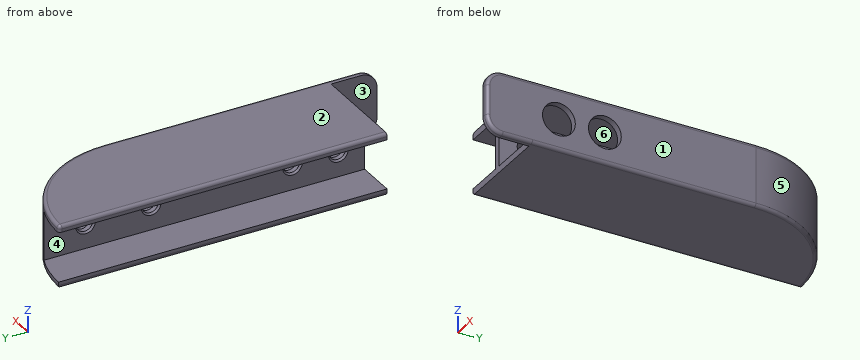
from build123d import *

# Parameters (mm, degrees)
BOSS_EXTRUDE1_DEPTH = 19
SKETCH2_W           = 24
SKETCH2_H           = 15
CUT_EXTRUDE1_DEPTH  = 29
SKETCH2_2_W         = 24
SKETCH2_2_H         = 15
CUT_EXTRUDE2_DEPTH  = 109
SHELL2_START        = 2
SHELL2_DEPTH        = 15
FILLET1_R           = 1
SKETCH8_W           = 2
SKETCH8_H           = 19
BOSS_EXTRUDE2_DEPTH = 14
FILLET3_R           = 5
FILLET4_R           = 1


# Read off the part's stored shape, not the designer's step: Shell2, M6 Tapped Hole1, Ø10.0mm Dowel Hole1
with BuildPart() as part:
    # Sketch1 → Boss-Extrude1 (new body)
    with BuildSketch(Plane.XY):
        with BuildLine():
            Line((32, 0), (32, 68))
            ThreePointArc((32, 68), (22.627416998, 90.627416998), (0, 100))
            Line((0, 100), (0, 0))
            Line((0, 0), (32, 0))
        make_face()
    extrude(amount=BOSS_EXTRUDE1_DEPTH)

    # Sketch2 → Cut-Extrude1 (cut)
    with BuildSketch(Plane(origin=(0, 0, 0), x_dir=(1, 0, 0), z_dir=(0, 1, 0))):
        with Locations((0, -9.5)):
            Rectangle(SKETCH2_W, SKETCH2_H)
    extrude(amount=CUT_EXTRUDE1_DEPTH, mode=Mode.SUBTRACT)

    # Sketch2<2> → Cut-Extrude2 (cut)
    with BuildSketch(Plane(origin=(0, 0, 0), x_dir=(1, 0, 0), z_dir=(0, 1, 0))):
        with Locations((0, -9.5)):
            Rectangle(SKETCH2_2_W, SKETCH2_2_H)
    extrude(amount=CUT_EXTRUDE2_DEPTH, mode=Mode.SUBTRACT)

    # Shell2 outline → Shell2 (cut)
    with BuildSketch(Plane.XY.offset(SHELL2_START)):
        with BuildLine():
            ThreePointArc((30, 68), (25.690465157, 83.491933385), (14, 94.532998323))
            Line((14, 94.532998323), (14, 0))
            Line((14, 0), (30, 0))
            Line((30, 0), (30, 68))
        make_face()
    extrude(amount=SHELL2_DEPTH, mode=Mode.SUBTRACT)

    # M6 Tapped Hole1 outline → M6 Tapped Hole1 (revolve, cut)
    with BuildSketch(Plane(origin=(0, 85, 9.5), x_dir=(0, 1, 0), z_dir=(0, 0, -1))):
        Polygon((2.5, 12.525), (2.5, 14), (0, 14), (0, 12), (3.025, 12), align=None)
    revolve(axis=Axis((0, 85, 9.5), (1, 0, 0)), mode=Mode.SUBTRACT)

    # M6 Tapped Hole1 2 outline → M6 Tapped Hole1 2 (revolve, cut)
    with BuildSketch(Plane(origin=(0, 65, 9.5), x_dir=(0, 1, 0), z_dir=(0, 0, -1))):
        Polygon((2.5, 12.525), (2.5, 14), (0, 14), (0, 12), (3.025, 12), align=None)
    revolve(axis=Axis((0, 65, 9.5), (1, 0, 0)), mode=Mode.SUBTRACT)

    # M6 Tapped Hole1 3 outline → M6 Tapped Hole1 3 (revolve, cut)
    with BuildSketch(Plane(origin=(0, 8, 9.5), x_dir=(0, 1, 0), z_dir=(0, 0, -1))):
        Polygon((2.5, 12.525), (2.5, 14), (0, 14), (0, 12), (3.025, 12), align=None)
    revolve(axis=Axis((0, 8, 9.5), (1, 0, 0)), mode=Mode.SUBTRACT)

    # M6 Tapped Hole1 4 outline → M6 Tapped Hole1 4 (revolve, cut)
    with BuildSketch(Plane(origin=(0, 22, 9.5), x_dir=(0, 1, 0), z_dir=(0, 0, -1))):
        Polygon((2.5, 12.525), (2.5, 14), (0, 14), (0, 12), (3.025, 12), align=None)
    revolve(axis=Axis((0, 22, 9.5), (1, 0, 0)), mode=Mode.SUBTRACT)

    # Ø10.0mm Dowel Hole1 outline → Ø10.0mm Dowel Hole1 (revolve, cut)
    with BuildSketch(Plane(origin=(0, 8, 9.5), x_dir=(0, 1, 0), z_dir=(0, 0, -1))):
        Polygon((5, 30.025), (5, 32), (0, 32), (0, 30), (5.025, 30), align=None)
    revolve(axis=Axis((0, 8, 9.5), (1, 0, 0)), mode=Mode.SUBTRACT)

    # 10.0mm Dowel Hole1 2 outline → 10.0mm Dowel Hole1 2 (revolve, cut)
    with BuildSketch(Plane(origin=(0, 22, 9.5), x_dir=(0, 1, 0), z_dir=(0, 0, -1))):
        Polygon((5, 30.025), (5, 32), (0, 32), (0, 30), (5.025, 30), align=None)
    revolve(axis=Axis((0, 22, 9.5), (1, 0, 0)), mode=Mode.SUBTRACT)

    # Fillet1
    fillet1_edges = [part.edges().sort_by_distance(p)[0] for p in [
        (22.627416998, 90.627416998, 19),
        (0, 50, 19),
        (0, 50, 0),
        (22.627416998, 90.627416998, 0),
        (32, 34, 0),
        (0, 100, 18),
        (32, 34, 19),
    ]]
    fillet(fillet1_edges, radius=FILLET1_R)

    # Sketch8 → Boss-Extrude2 (add)
    with BuildSketch(Plane(origin=(0, 0, 0), x_dir=(1, 0, 0), z_dir=(0, 1, 0))):
        with Locations((31, -9.5)):
            Rectangle(SKETCH8_W, SKETCH8_H)
    extrude(amount=-BOSS_EXTRUDE2_DEPTH)

    # Fillet3
    fillet3_edges = [part.edges().sort_by_distance(p)[0] for p in [
        (31, -14, 19),
        (31, -14, 0),
    ]]
    fillet(fillet3_edges, radius=FILLET3_R)

    # Fillet4
    fillet4_edges = [part.edges().sort_by_distance(p)[0] for p in [
        (32, -12.535533906, 1.464466094),
        (32, -14, 9.5),
        (32, -12.535533906, 17.535533906),
        (32, -4.5, 0),
        (32, -4.5, 19),
    ]]
    fillet(fillet4_edges, radius=FILLET4_R)


solid = part.part
Work out the finished part from the listing and answer in its coordinate system (mm). Face numbers are marked on the shaded views. A direction names the side the tool comes from. Coordinates: 2 decimals unless noted, no trailing zeros. Write each loop counter-clockwise with the first axis right and the second up, starting at its lowest first coordinate (ties: lowest second). Pieces come first, ordered by that corner, then holes. Notation, with made-up numbers: M 34,54.5 L 54,54.5 A29 cw 54,88.5 Z; hole C 76,19.25 d2. An arc over 180 degrees is marked long. Answer as CSV lines item,"result". Start each with the question number.
Item 1: Section A-A on y = 8 is taken. Write down the section's boundary in (x, z) (3 decimals), and give its area (3 significant figures).
Item 2: Section B-B on y = 56.5 is taken. Write down the section's boundary in (x, z), and give its area (3 significant figures).
Item 3: A tool of negligible diameter and unlimited length cuts with its end or side. For the marked faces 4, 5 and 6, from which of +Z, -Z, +X, -X, +Y, -Y can it reach the whole face along a straight path? Write none if from no direction.
Item 4: Section C-C on z = 9.5 is taken. Give the number of separate pieces and of enclosed holes in the cut face, and give its area (3 significant figures).
Item 5: Determine the mould class of the marked faces 1, 2 and 3 for opening direction X: released by +X, released by -X, zero draft, split by the parting line, or undercut.
Item 6: Flat-ended cylindrical pins translate along their axes: P1, Ø5.5, axis at x = 13.5, z = 11, coming from the -Y side; P2, Ø8, axis at y = 8, z = 9.5, coming from the -X side; P3, Ø9, axis at y = 8, z = 9.5, coming from the +X side; P4, Ø5, axis at x = 6.5, z = 5.5, coming from the -Y side. Find the tip coordinate at first contact, or state that the pin passes through.
Item 7: Consider L1, parallel to Z at x = 13, y = 85; L2, parallel to Z at x = 29.5, y = 8.5; L3, parallel to X at y = 23.5, z = 15. Determine where each line is inside the solid, lowest interval first.
Checks:
1,outline,"M 0,1 A1 ccw 1,0 L 31,0 A1 ccw 32,1 L 32,4.5 L 30.025,4.5 L 30,4.475 L 30,2 L 14,2 L 14,7 L 12.525,7 L 12,6.475 L 12,2 L 0,2 Z; M 0,17 L 12,17 L 12,12.525 L 12.525,12 L 14,12 L 14,17 L 30,17 L 30,14.525 L 30.025,14.5 L 32,14.5 L 32,18 A1 ccw 31,19 L 1,19 A1 ccw 0,18 Z"
1,area,"157 mm²"
2,outline,"M 0,1 A1 ccw 1,0 L 31,0 A1 ccw 32,1 L 32,18 A1 ccw 31,19 L 1,19 A1 ccw 0,18 L 0,17 L 12,17 L 12,2 L 0,2 Z; hole M 14,2 L 30,2 L 30,17 L 14,17 Z"
2,area,"187 mm²"
3,face 4,"-X, +Y, -Y"
3,face 5,"+Z, -Z, +X, +Y"
3,face 6,"-Y"
4,separate pieces,"7"
4,enclosed holes,"0"
4,area,"345 mm²"
5,face 1,"released by +X"
5,face 2,"zero draft"
5,face 3,"undercut"
6,P1,"stops at y = 0"
6,P2,"stops at x = 12"
6,P3,"stops at x = 14"
6,P4,"passes through"
7,L1,"z = 0 to 7, 12 to 19"
7,L2,"z = 0 to 2, 17 to 19"
7,L3,"x = 12 to 14, 30 to 32"
